Can you work these out from the model? Positions are in its coordinate system, mm. Round coordinates to 2 decimals unless told otherwise and drop trailing zeros. Loops run counter-clockwise (first coordinate to the right, second up) from the corner with the lowest first, then second, coordinate; pieces in that order, holes last. Notation, with made-up numbers: M -26.5,84 L -7.5,84 A26 ccw -7.5,123 Z; hole C 8,62 d6. An arc over 180 degrees is marked long. Return JSON: item names as keys, results as strings.
```python
from build123d import *

# Parameters (mm, degrees)
SKETCH1_W           = 150
SKETCH1_H           = 44.45
BOSS_EXTRUDE1_DEPTH = 6
SKETCH2_R           = 3.666174209
CUT_EXTRUDE1_DEPTH  = 157.562455589
SKETCH3_R           = 3.175
CUT_EXTRUDE2_DEPTH  = 157.562455589


with BuildPart() as part:
    # Sketch1 → Boss-Extrude1 (new body)
    with BuildSketch(Plane.XY):
        with Locations((75, 22.225)):
            Rectangle(SKETCH1_W, SKETCH1_H)
    extrude(amount=BOSS_EXTRUDE1_DEPTH)

    # Sketch2 → Cut-Extrude1 (cut, through all)
    with BuildSketch(Plane.XY.offset(6)):
        with Locations((11.495, 22.225)):
            Circle(SKETCH2_R)
        with Locations(Location((138.505, 22.225, 0), (0, 0, 180))):
            Circle(SKETCH2_R)
    extrude(amount=-CUT_EXTRUDE1_DEPTH, mode=Mode.SUBTRACT)

    # Sketch3 → Cut-Extrude2 (cut, through all)
    with BuildSketch(Plane(origin=(0, 0, 0), x_dir=(-1, 0, 0), z_dir=(0, 0, -1))):
        with Locations((-75, 7.62)):
            Circle(SKETCH3_R)
        with Locations((-75, 34.197995036)):
            Circle(SKETCH3_R)
    extrude(amount=-CUT_EXTRUDE2_DEPTH, mode=Mode.SUBTRACT)


solid = part.part
```
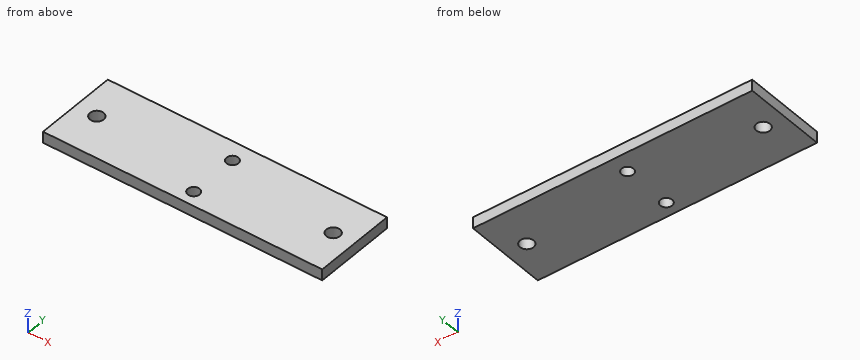
Q1. Suppose I cut it at C-C, the plane x = 139.5. Please give me the cut outline in (y, z).
Results:
{"outline": "M 0,0 L 18.7,0 L 18.7,6 L 0,6 Z; M 25.75,0 L 44.45,0 L 44.45,6 L 25.75,6 Z"}
Q2. I'm going to push a flat-ended pin straight in: pin 1 Ø11.5 at (x, y) = (11.495, 22.225) entering from -Z. Where does the tip first touch, or does it pass through?
Results:
{"pin 1": "stops at z = 0"}
Q3. If I drill on line 1 along X through (y, z) = (21, 2.3); line 2 along X through (y, z) = (19, 4.1); line 3 along X through (y, z) = (10, 3.5), over which ranges is the centre line in solid material (lowest first)?
Results:
{"line 1": "x = 0 to 8.04, 14.95 to 135.05, 141.96 to 150", "line 2": "x = 0 to 9.75, 13.24 to 136.76, 140.25 to 150", "line 3": "x = 0 to 72.9, 77.1 to 150"}
Q4. Suppose I cut it at A-A, the plane x = 75. Please give me the cut outline in (y, z) (3 decimals).
Results:
{"outline": "M 0,0 L 4.445,0 L 4.445,6 L 0,6 Z; M 10.795,0 L 31.023,0 L 31.023,6 L 10.795,6 Z; M 37.373,0 L 44.45,0 L 44.45,6 L 37.373,6 Z"}
Q5. Suppose I cut it at D-D, the plane z = 2.2. Please give me the cut outline in (x, y) (3 decimals).
Results:
{"outline": "M 0,0 L 150,0 L 150,44.45 L 0,44.45 Z; hole C 11.495,22.225 d7.332; hole C 75,7.62 d6.35; hole C 75,34.198 d6.35; hole C 138.505,22.225 d7.332"}
Q6. Suppose I cut it at B-B, the plane y = 7.62. Please give me the cut outline in (x, z) (3 decimals), plus the area to 3 significant figures.
Results:
{"outline": "M 0,0 L 71.825,0 L 71.825,6 L 0,6 Z; M 78.175,0 L 150,0 L 150,6 L 78.175,6 Z", "area": "862 mm2"}
